from build123d import *

# Parameters (mm, degrees)
F1_DEPTH = 25


with BuildPart() as f1:
    # F0 (on Top) → F1 (new body)
    with BuildSketch(Plane.XY):
        Polygon((30.266396, -8.176231), (8.176231, 30.266396), (-30.266396, 8.176231), (-8.176231, -30.266396), align=None)
    extrude(amount=F1_DEPTH)

    # F1_face (on face) → F4 section 0
    with BuildSketch(Plane.XY.offset(25), mode=Mode.PRIVATE) as f4_s0:
        Polygon((-8.176231, -30.266396), (30.266396, -8.176231), (8.176231, 30.266396), (-30.266396, 8.176231), align=None)
    loft([f4_s0.sketch, Vertex(0, 0, 150)])


solid = f1.part
For this review, take the finished solid that the model builds, in its own axes (mm). Round coordinates to 2 decimals unless told otherwise and drop trailing zeros. Order: outer loops, then holes, each group sorted by start corner. A loop starts at its lowest first (then second) coordinate and runs counter-clockwise, first axis right, second up. Notation, with made-up numbers: M 2.5,-29 L 45.5,-29 A20 cw 45.5,1 Z; hole C -32,18.5 d1. An arc over 180 degrees is marked long. Use a Markdown table: item, result. Add a question column.
Item 1: To check wall thickness, follow line 1 along Y through (x, z) = (-21.5, 60); line 2 along X through (y, z) = (-2, 128.5); line 3 along Y through (x, z) = (0.5, 75.5). State the ranges of each line that lie inside material, in increasing order.
Item 2: Add section A-A, the plane y = 15.5. Give the boundary of the cut face in (x, z), then the cut area to 3 significant figures.
Item 3: Insertion check: pin 1 (5 mm diameter, centred on y = 10, z = 85.5, fed in from -X); pin 2 (5 mm diameter, centred on y = -1, z = 36, fed in from +X); pin 3 (12 mm diameter, centred on x = -8.5, z = 92.5, fed in from +Y). Each pin has a flat end and moves straight along its axis. Give the tip position at first contact, or say it passes through.
Item 4: Add section D-D, the plane y = 5. Give the boundary of the cut face in (x, z).
Item 5: Add section C-C, the plane z = 100. Give the boundary of the cut face in (x, y), then the cut area to 3 significant figures.
Item 6: Add section B-B, the plane x = -16.5. Give the boundary of the cut face in (y, z).
Geometry results:
| question | item | result |
|---|---|---|
| 1 | line 1 | y = 5.38 to 6.05 |
| 1 | line 2 | x = -3.25 to 4.17 |
| 1 | line 3 | y = -14.95 to 15.53 |
| 2 | outline | M -17.52,0 L 16.66,0 L 16.66,25 L 4.19,85.99 L -17.52,25 Z |
| 2 | area | 1,900 mm² |
| 3 | pin 1 | stops at x = -10 |
| 3 | pin 2 | stops at x = 25.42 |
| 3 | pin 3 | stops at y = 10.54 |
| 4 | outline | M -28.44,0 L 22.69,0 L 22.69,25 L 1.35,129.35 L -18.51,73.56 L -28.44,25 Z |
| 5 | outline | M -12.11,3.27 L -3.27,-12.11 L 12.11,-3.27 L 3.27,12.11 Z |
| 5 | area | 315 mm² |
| 6 | outline | M -15.78,0 L 16.09,0 L 16.09,25 L 4.46,81.86 L -15.78,25 Z |
